from build123d import *

# Parameters (mm, degrees)
F0_R     = 12.5
F1_DEPTH = 8
F2_SIZE  = 1


with BuildPart() as f1:
    # F0 (on Front) → F1 (new body, symmetric)
    with BuildSketch(Plane.XZ):
        with BuildLine():
            Line((-75, 10.5947501931), (-75, -47.5))
            Line((-75, -47.5), (75, -47.5))
            Line((75, -47.5), (75, 10.5947501931))
            ThreePointArc((75, 10.5947501931), (73.3711730709, 18.5004443435), (68.75, 25.1184377414))
            ThreePointArc((68.75, 25.1184377414), (0, 52.5), (-68.75, 25.1184377414))
            ThreePointArc((-68.75, 25.1184377414), (-73.3711730709, 18.5004443435), (-75, 10.5947501931))
        make_face()
        Circle(F0_R, mode=Mode.SUBTRACT)
    extrude(amount=F1_DEPTH, both=True)

    # F2
    f2_edges = [f1.edges().sort_by_distance(p)[0] for p in [
        (-12.5, -8, 0),
        (-12.5, 8, 0),
    ]]
    chamfer(f2_edges, length=F2_SIZE)


solid = f1.part
Input: part model. Units: mm. Frame: model coordinates. Coordinates: 2 decimals unless noted, no trailing zeros. Loops run counter-clockwise (first coordinate to the right, second up) from the corner with the lowest first, then second, coordinate; pieces in that order, holes last.
(1) First-contact query: pin 1 Ø6 at (x, y) = (-60, 1) entering from +Z; pin 2 Ø2 at (y, z) = (1.5, 30.5) entering from -X; pin 3 Ø8 at (y, z) = (5, 29.5) entering from -X. Flat tips, straight axial feed; report the tip coordinate or a pass-through.
(2) Section D-D on x = -20. Return the cut outline in (y, z), then the cut area to 3 significant figures.
(3) Section B-B on x = 0. Return the cut outline in (y, z).
(4) Section A-A on z = 0. Return the cut outline in (x, y), then the cut area to 3 significant figures.
(5) Material intervals for probe 1 along Z at (x, y) = (0, 3.25); probe 2 along Z at (x, y) = (-6.5, 4.25); probe 3 along X at (y, z) = (-4.75, 11), sorted ascending.
(6) Section C-C on y = -2.75. Return the cut outline in (x, z).
(7) Pull-direction query (X, two-part tool) for faces 1 (the face through (-1, 0, -47.5)), 2 (the face through (-75, 0, -18)), 3 (the face through (11.923, 0.098, 3.755)); classes: released by +X, released by -X, zero draft, split by the parting line, or undercut.
Data:
1. pin 1: stops at z = 34.66
1. pin 2: stops at x = -63.8
1. pin 3: stops at x = -68.34
2. outline: (-8, -47.5) - (8, -47.5) - (8, 50.48) - (-8, 50.48) - close
2. area: 1,570 mm2
3. outline: (-8, -47.5) - (8, -47.5) - (8, -13.5) - (7, -12.5) - (-7, -12.5) - (-8, -13.5) - close; (-8, 13.5) - (-7, 12.5) - (7, 12.5) - (8, 13.5) - (8, 52.5) - (-8, 52.5) - close
4. outline: (-75, -8) - (-13.5, -8) - (-12.5, -7) - (-12.5, 7) - (-13.5, 8) - (-75, 8) - close; (12.5, -7) - (13.5, -8) - (75, -8) - (75, 8) - (13.5, 8) - (12.5, 7) - close
4. area: 2,000 mm2
5. probe 1: z = -47.5 to -12.5, 12.5 to 52.5
5. probe 2: z = -47.5 to -10.68, 10.68 to 52.29
5. probe 3: x = -75 to -5.94, 5.94 to 75
6. outline: (-75, -47.5) - (75, -47.5) - (75, 10.59) arc R20 ccw to (68.75, 25.12) arc R100 ccw to (-68.75, 25.12) arc R20 ccw to (-75, 10.59) - close; hole circle Ø25 at (0, 0)
7. face 1: zero draft
7. face 2: released by -X
7. face 3: undercut
